Verification items for the finished model (mm, model axes). Face numbers are marked on the shaded views. A direction names the side the tool comes from. Coordinates: 2 decimals unless noted, no trailing zeros. Write each loop counter-clockwise with the first axis right and the second up, starting at its lowest first coordinate (ties: lowest second). Pieces come first, ordered by that corner, then holes. Notation, with made-up numbers: (31.25, 61) -> (38.25, 61) arc R22 ccw to (38.25, 78) -> close; hole circle Ø9 at (87, 9.5). An arc over 180 degrees is marked (long way). Write item = value, one per line. Start each with the question number.
(1) Material ranges on probe 1 along X at (y, z) = (-15, 42); probe 2 along X at (y, z) = (-63.5, 30.5); probe 3 along Z at (x, y) = (-60, -42), recorded low to high. Write a range as [from, to].
(2) Section check C-C (x = -26). Record the cut outline in (y, z).
(3) Section check A-A (z = 3). Record the cut outline in (x, y).
(4) Gauge pin test, flat ends, axial feed: pin 1 Ø19.5 at (x, y) = (-75, -44.5) entering from +Z; pin 2 Ø3 at (y, z) = (-46, 36.5) entering from -X. Record the tip position at first contact, or that the pin passes through.
(5) Section check D-D (x = -68.5). Record the cut outline in (y, z), plus the area to 3 significant figures.
(6) Mould release check, pull along X, two halves, no side actions. Record for the marked faces 1, 2 and 3: released by +X, released by -X, zero draft, split by the parting line, or undercut.
(7) Set-up check for the marked faces 4, 5 and 6: record each of +Z, -Z, +X, -X, +Y, -Y from which the full face is reachable in a straight line by a thin tool's end or side.
(8) Section check B-B (y = -43). Record the cut outline in (x, z).
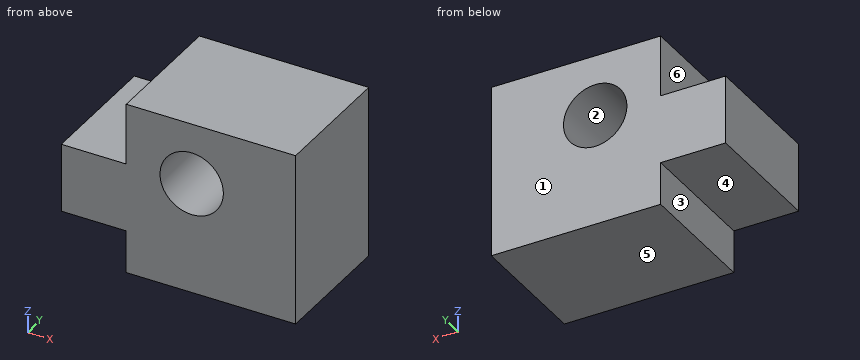
```python
from build123d import *

# Parameters (mm, degrees)
F1_DEPTH = 76.2
F2_R     = 18.84371
F3_DEPTH = 76.2


with BuildPart() as f1:
    # F0 (on Front) → F1 (new body)
    with BuildSketch(Plane.XZ):
        Polygon((-57.544138, 17.34207), (-96.169658, 17.34207), (-96.169658, -23.451207), (-57.544138, -23.451207), (-57.544138, -48.873104), (43.158107, -48.873104), (43.158107, 53.799827), (-57.544138, 53.799827), align=None)
    extrude(amount=F1_DEPTH)

    # F2 (on face) → F3 (cut)
    with BuildSketch(Plane.XZ.offset(76.2)):
        with Locations((-18.626319, 17.434625)):
            Circle(F2_R)
    extrude(amount=-F3_DEPTH, mode=Mode.SUBTRACT)


solid = f1.part
```
Response:
q1.probe_1 = [-57.54, 43.16]
q1.probe_2 = [-57.54, -32.21], [-5.05, 43.16]
q1.probe_3 = [-23.45, 17.34]
q2.outline = (-76.2, -48.87) -> (0, -48.87) -> (0, 0.09) -> (-76.2, 0.09) -> close; (-76.2, 34.78) -> (0, 34.78) -> (0, 53.8) -> (-76.2, 53.8) -> close
q3.outline = (-96.17, -76.2) -> (-30.74, -76.2) -> (-30.74, 0) -> (-96.17, 0) -> close; (-6.51, -76.2) -> (43.16, -76.2) -> (43.16, 0) -> (-6.51, 0) -> close
q4.pin_1 = 17.34
q4.pin_2 = -57.54
q5.outline = (-76.2, -23.45) -> (0, -23.45) -> (0, 17.34) -> (-76.2, 17.34) -> close
q5.area = 3,110 mm2
q6.face_1 = zero draft
q6.face_2 = undercut
q6.face_3 = released by -X
q7.face_4 = -Z, -X, +Y, -Y
q7.face_5 = -Z, +X, -X, +Y, -Y
q7.face_6 = +Z, -X, +Y, -Y
q8.outline = (-96.17, -23.45) -> (-57.54, -23.45) -> (-57.54, -48.87) -> (43.16, -48.87) -> (43.16, 53.8) -> (-57.54, 53.8) -> (-57.54, 17.34) -> (-96.17, 17.34) -> close; hole circle Ø37.69 at (-18.63, 17.43)
